Input: part model. Units: mm. Frame: model coordinates. Coordinates: 2 decimals unless noted, no trailing zeros. Order: outer loops, then holes, each group sorted by start corner. A loop starts at its lowest first (then second) coordinate and runs counter-clockwise, first axis right, second up.
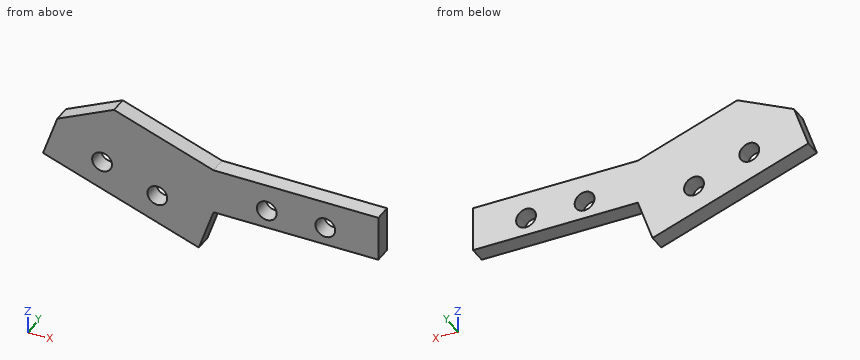
from build123d import *

# Parameters (mm, degrees)
SKETCH2_W           = 29.13019228
SKETCH2_H           = 8.0032651
BOSS_EXTRUDE1_DEPTH = 3
SKETCH3_R           = 1.75
CUT_EXTRUDE1_DEPTH  = 3
SKETCH5_W           = 29.13
SKETCH5_H           = 3
BOSS_EXTRUDE2_DEPTH = 8
SKETCH6_R           = 1.75
CUT_EXTRUDE3_DEPTH  = 7
CUT_EXTRUDE4_DEPTH  = 5
CUT_EXTRUDE5_DEPTH  = 3
CUT_EXTRUDE7_DEPTH  = 10


with BuildPart() as part:
    # Sketch2 → Boss-Extrude1 (new body)
    with BuildSketch(Plane(origin=(0, 0, 0), x_dir=(1, 0, 0), z_dir=(0, 1, 0))):
        Polygon((-50.225743969, 28.670443259), (-77.768700077, 19.18664292), (-77.768700077, 11.18337782), (-50.225743969, 20.667178159), align=None)
        with Locations((-35.660647829, 24.668810709)):
            Rectangle(SKETCH2_W, SKETCH2_H)
    extrude(amount=BOSS_EXTRUDE1_DEPTH)

    # Sketch3 → Cut-Extrude1 (cut)
    with BuildSketch(Plane.XZ):
        with Locations(Location((-30.470551689, -25.467178146, 0), (0, 0, 270))):
            Circle(SKETCH3_R)
        with Locations(Location((-40.820551689, -25.467178146, 0), (0, 0, 270))):
            Circle(SKETCH3_R)
    extrude(amount=-CUT_EXTRUDE1_DEPTH, mode=Mode.SUBTRACT)

    # Sketch5 → Boss-Extrude2 (add)
    with BuildSketch(Plane(origin=(-14.149302504, 0, -41.092558245), x_dir=(-0.9455185755993176, 0, 0.32556815445715426), z_dir=(-0.32556815445715426, 0, -0.9455185755993176))):
        with Locations((52.720190597, 1.5)):
            Rectangle(SKETCH5_W, SKETCH5_H)
    extrude(amount=BOSS_EXTRUDE2_DEPTH)

    # Sketch6 → Cut-Extrude3 (cut)
    with BuildSketch(Plane.XZ):
        with Locations(Location((-69.935655683, -25.201370089, 0), (0, 0, 270))):
            Circle(SKETCH6_R)
        with Locations(Location((-60.159815933, -28.600701946, 0), (0, 0, 270))):
            Circle(SKETCH6_R)
    extrude(amount=-CUT_EXTRUDE3_DEPTH, mode=Mode.SUBTRACT)

    # Sketch7 → Cut-Extrude4 (cut)
    with BuildSketch(Plane.XZ):
        Polygon((-77.768700077, -19.18664292), (-75.305049077, -12.031680889), (-77.768700077, -11.18337782), align=None)
    extrude(amount=-CUT_EXTRUDE4_DEPTH, mode=Mode.SUBTRACT)

    # Sketch9 → Cut-Extrude5 (cut)
    with BuildSketch(Plane.XZ):
        with BuildLine():
            Line((-75.305049077, -12.031680889), (-77.847985202, -19.416903645))
            add(Edge.make_bspline(
                [(-69.0352228, -14.190555206), (-74.086749011, -15.68616926), (-77.847985202, -19.416903645)],
                knots=[0, 0, 0, 1, 1, 1], degree=2))
            Line((-69.0352228, -14.190555206), (-75.305049077, -12.031680889))
        make_face()
    extrude(amount=-CUT_EXTRUDE5_DEPTH, mode=Mode.SUBTRACT)

    # Sketch10 → Cut-Extrude7 (cut)
    with BuildSketch(Plane.XZ):
        with BuildLine():
            Line((-75.305049077, -12.031680889), (-77.847985202, -19.416903645))
            add(Edge.make_bspline(
                [(-69.0352228, -14.190555206), (-74.086749011, -15.68616926), (-77.847985202, -19.416903645)],
                knots=[0, 0, 0, 1, 1, 1], degree=2))
            Line((-69.0352228, -14.190555206), (-75.305049077, -12.031680889))
        make_face()
        with BuildLine():
            add(Edge.make_bspline(
                [(-69.0352228, -14.190555206), (-74.086749011, -15.68616926), (-77.847985202, -19.416903645)],
                knots=[0, 0, 0, 1, 1, 1], degree=2))
            Line((-77.847985202, -19.416903645), (-67.8223159, -14.608192544))
            Line((-67.8223159, -14.608192544), (-69.0352228, -14.190555206))
        make_face()
    extrude(amount=-CUT_EXTRUDE7_DEPTH, mode=Mode.SUBTRACT)


solid = part.part
Item 1: Cut plane A-A on z = -25. Return loops of the section in (x, y).
Response values:
outline: (-79.77, 0) - (-71.67, 0) - (-71.67, 3) - (-79.77, 3) - close; (-68.2, 0) - (-42.51, 0) - (-42.51, 3) - (-68.2, 3) - close; (-39.13, 0) - (-32.16, 0) - (-32.16, 3) - (-39.13, 3) - close; (-28.78, 0) - (-21.1, 0) - (-21.1, 3) - (-28.78, 3) - close
Item 2: Pin query (flat end, axial travel): pin 1 Ø12 at (x, z) = (-45.5, -17.5) entering from -Y; pin 2 Ø1.5 at (y, z) = (0.5, -17) entering from -X; pin 3 Ø3 at (x, z) = (-69.94, -25.2) entering from -Y; pin 4 Ø1.5 at (x, y) = (-59, 1.5) entering from -Z. Return the tip coordinate at first contact, or that it passes through.
Response values:
pin 1: stops at y = 0
pin 2: stops at x = -74.37
pin 3: passes through
pin 4: stops at z = -34.37
Item 3: Ray query, probe 1 along X at (y, z) = (1.7, -25.5); probe 2 along X at (y, z) = (2.1, -25); probe 3 along Z at (x, y) = (-24, 2.5). Return the intervals inside material, ascending.
Response values:
probe 1: x = -79.94 to -71.66, -68.21 to -42.57, -39.07 to -32.22, -28.72 to -21.1
probe 2: x = -79.77 to -71.67, -68.2 to -42.51, -39.13 to -32.16, -28.78 to -21.1
probe 3: z = -28.67 to -20.67
Item 4: Cut plane B-B on y = 1.3. Return loops of the section in (x, z).
Response values:
outline: (-80.37, -26.75) - (-52.83, -36.23) - (-50.23, -28.67) - (-21.1, -28.67) - (-21.1, -20.67) - (-50.23, -20.67) - (-67.82, -14.61) - (-77.85, -19.42) - close; hole circle Ø3.5 at (-69.94, -25.2); hole circle Ø3.5 at (-60.16, -28.6); hole circle Ø3.5 at (-40.82, -25.47); hole circle Ø3.5 at (-30.47, -25.47)
Item 5: Cut plane D-D on z = -22.5. Return loops of the section in (x, y), then the cut area to 3 significant figures.
Response values:
outline: (-78.91, 0) - (-21.1, 0) - (-21.1, 3) - (-78.91, 3) - close
area: 173 mm2
Item 6: Cut plane C-C on x = -25. Return loops of the section in (y, z), then the cut area to 3 significant figures.
Response values:
outline: (0, -28.67) - (3, -28.67) - (3, -20.67) - (0, -20.67) - close
area: 24.0 mm2
